Input: dimensioned drawing with shaded views. Units: mm. Origin: part minimum x, y, z. Coordinates: 2 decimals unless noted, no trailing zeros. Order: outer loops, then holes, each group sorted by start corner. A loop starts at its lowest first (then second) coordinate and runs counter-clockwise, first axis right, second up. Notation, with made-up numbers: M -29.75,87.25 L -19.75,87.25 A19 ccw -19.75,96.25 Z; hole C -15.5,-35 d3. An arc over 180 degrees is marked long. Use CSV: the item, a comma, the result in double quotes. Start each with the question number.
1. First-contact query: P1, Ø6, axis at x = 18.5, z = 319.5, coming from the +Y side; P2, Ø5, axis at x = 4, z = 168, coming from the -Y side; P3, Ø6, axis at y = 8.5, z = 193, coming from the -X side. Flat tips, straight axial feed; report the tip coordinate or a pass-through.
2. Material intervals for line 1 (Y direction, x = 16, z = 217); line 2 (Y direction, x = 16.25, z = 359); line 3 (X direction, y = 4.25, z = 550), sorted ascending.
3. Section query A-A on z = 269.5. Return the cut outline in (x, y).
4. Section query C-C on x = 6.75. Return the cut outline in (y, z).
5. Section query B-B on y = 4.75. Return the cut outline in (x, z).
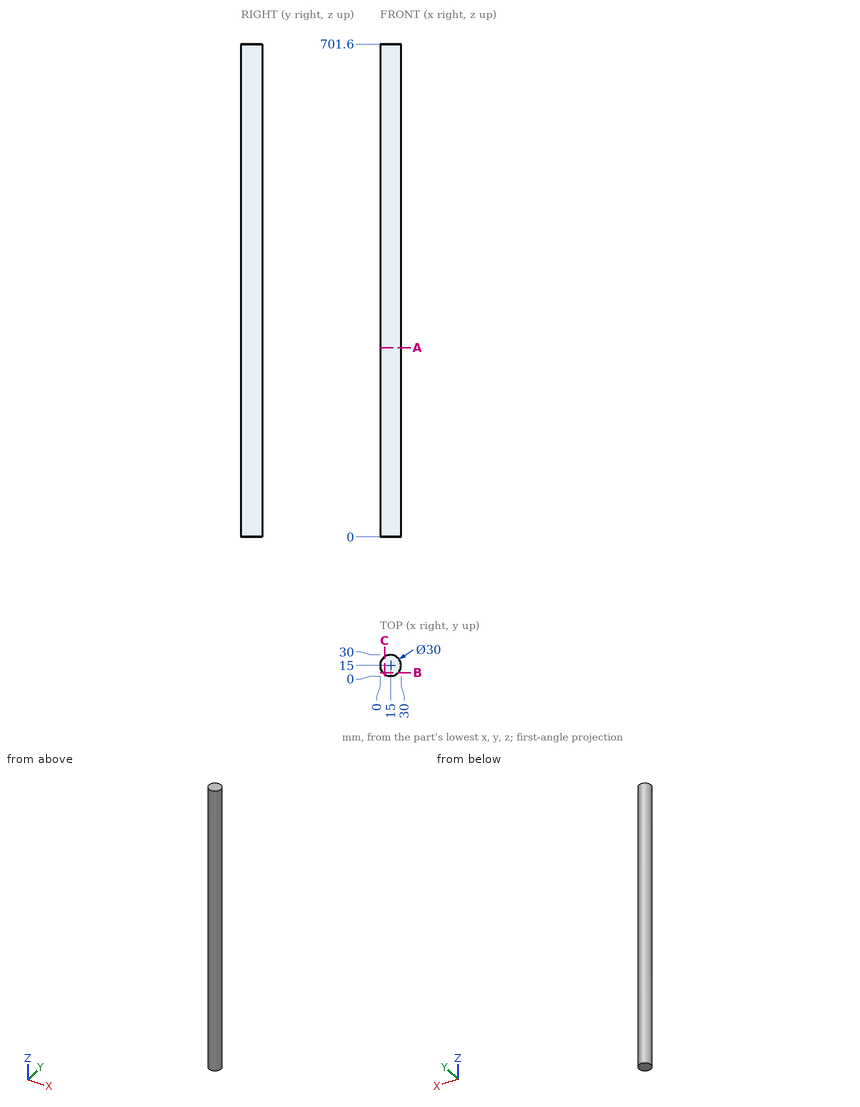
Results list:
1,P1,"stops at y = 29.99"
1,P2,"stops at y = 2.64"
1,P3,"stops at x = 0.41"
2,line 1,"y = 0.03 to 29.97"
2,line 2,"y = 0.05 to 29.95"
2,line 3,"x = 4.54 to 25.46"
3,outline,"C 15,15 d30"
4,outline,"M 2.47,0 L 27.53,0 L 27.53,701.6 L 2.47,701.6 Z"
5,outline,"M 4.05,0 L 25.95,0 L 25.95,701.6 L 4.05,701.6 Z"
